from build123d import *

# Parameters (mm, degrees)
F1_DEPTH = 1155.7
F3_D     = 13.49248


with BuildPart() as f1:
    # F0 (on Front) → F1 (new body)
    with BuildSketch(Plane.XZ):
        Polygon((0, 101.6), (0, 0), (50.8, 0), (50.8, 3.175), (3.175, 3.175), (3.175, 101.6), align=None)
    extrude(amount=F1_DEPTH)

    # F3 (through all)
    with Locations(Plane.XY.offset(3.175)):
        with Locations((26.9875, -577.85), (26.9875, -196.85), (26.9875, -958.85)):
            Hole(F3_D / 2)


solid = f1.part
Can you work these out from the model? Positions are in its coordinate system, mm. A direction names the side the tool comes from. Coordinates: 2 decimals unless noted, no trailing zeros. Loops run counter-clockwise (first coordinate to the right, second up) from the corner with the lowest first, then second, coordinate; pieces in that order, holes last. Notation, with made-up numbers: (46.5, 64.5) - (97.5, 64.5) arc R8 ccw to (97.5, 70.5) - close; hole circle Ø3 at (37, -34.5). An arc over 180 degrees is marked (long way). Answer as a JSON object with one key per item and string values. Group by question number.
Item 1: If we section it at C-C (z = 40.5): List the corners of the cut face in (x, y) for me (3 decimals), plus the area to 3 significant figures.
Item 2: If we section it at A-A (x = 12): List the corners of the cut face in (y, z) for me (3 decimals).
Item 3: If we section it at B-B (y = -939): List the corners of the cut face in (x, z) for me (3 decimals).
Item 4: On a 3-axis mill with a long thin cutter (end or side, diameter ignored), from which of +Z, -Z, +X, -X, +Y, -Y can I reach the whole of each face in a straight line? I mean faces 1 (the face through (25, -570, 0)), 2 (the face through (27, -570, 3.175)). Say none if no direction works.
Item 5: For pin 1 (4 mm diameter, centred on x = 42, y = -667, fed in from +Z) (3 decimals); pin 2 (10 mm diameter, centred on y = -859, z = 56, fed in from +X) (3 decimals), each with a flat end and sliding along its axis, tell me the tip position at first contact or that it passes through.
Item 6: If I drill on L1, parallel to X at y = -958.85, z = 1.9; L2, parallel to X at y = -958, z = 2; L3, parallel to X at y = -899, z = 16 (3 decimals), over which ranges is the centre line in solid material (lowest first)? Write a range as from..to.
Returned:
{
 "1": {"outline": "(0, -1155.7) - (3.175, -1155.7) - (3.175, 0) - (0, 0) - close", "area": "3,670 mm²"},
 "2": {"outline": "(-1155.7, 0) - (0, 0) - (0, 3.175) - (-1155.7, 3.175) - close"},
 "3": {"outline": "(0, 0) - (50.8, 0) - (50.8, 3.175) - (3.175, 3.175) - (3.175, 101.6) - (0, 101.6) - close"},
 "4": {"face 1": "-Z, +X, -X, +Y, -Y", "face 2": "+Z, +X, +Y, -Y"},
 "5": {"pin 1": "stops at z = 3.175", "pin 2": "stops at x = 3.175"},
 "6": {"L1": "x = 0..20.24, 33.73..50.8", "L2": "x = 0..20.3, 33.68..50.8", "L3": "x = 0..3.175"}
}
